Geometry check sheet. Reference: the model listing, model coordinates, mm. A direction names the side the tool comes from. Round coordinates to 2 decimals unless told otherwise and drop trailing zeros. Loops run counter-clockwise (first coordinate to the right, second up) from the corner with the lowest first, then second, coordinate; pieces in that order, holes last. Notation, with made-up numbers: (65, -6.5) - (98, -6.5) arc R14 ccw to (98, 20.5) - close; hole circle Ø4 at (49, 2.25). An arc over 180 degrees is marked (long way). Answer as CSV lines item,"result". Start each with the question number.
1) Cross-section at B-B on y = 27.5. Record the boundary of the cut face in (x, z).
2) Depth check by flat-ended pin: P1, Ø10, axis at y = 8.5, z = -25, coming from the +X side; P2, Ø3.5, axis at y = 14, z = 31, coming from the +X side; P3, Ø2, axis at x = -6.5, z = 17.5, coming from the +Y side; P4, Ø3.5, axis at x = 27, z = 22, coming from the +Y side. Enter the tip coordinate at first touch or a pass-through.
3) Cross-section at A-A on z = -22. State how many separate pieces and enclosed holes the cut face has, and give its area (3 significant figures).
4) Draft check along X on faces 1 (the cylindrical face through (-26.2, 1.23, 20.06)), 2 (the flat face through (0, 37, 30)), 3 (the flat face through (-29.98, 4.52, -29.87)). Enter one of: released by +X, released by -X, zero draft, split by the parting line, or undercut.
5) Cross-section at D-D on z = -1. Record the boundary of the cut face in (x, y), and give its area (3 significant figures).
6) Access from +Z, -Z, +X, -X, +Y, -Y to the whole of each face (thin tool, end or side, straight path). Record for faces 4 (the flat face through (13, 17, 39)), 5 (the flat face through (0, 36, 39)), 6 (the flat face through (0, 15, 20.65)), 7 (the flat face through (8, 15, 40)), 8 (the cylindrical face through (29.95, 4.27, -20.12)).
7) Thickness scan on line 1 along X through (y, z) = (0.65, -22); line 2 along Z through (x, y) = (-27, 1); line 3 along X through (y, z) = (9.5, 30). Record the ranges inside material, lowest first.
8) Cross-section at C-C on x = -19. Record the boundary of the cut face in (y, z).
from build123d import *

# Parameters (mm, degrees)
SKETCH1_R                          = 2.1
MAIN_CAP_EXTRUDE_DEPTH             = 6
MAIN_BODY_CHAMFER_SIZE             = 3
SKETCH4_R                          = 3.5
HOLE_COUNTERSINK_CUT_DEPTH         = 3
HOLE_COUNTERSINK_CHAMFER_SIZE      = 0.5
MAIN_PINION_CHIMNEY_EXTRUDE_DEPTH  = 32
SKETCH3_W                          = 28
SKETCH3_H                          = 24
PINION_CHIMNEY_CAP_EXTRUDE_DEPTH   = 5
INTERNAL_CHIMNEY_CHAMFER_SIZE      = 1
MAIN_CHIMNEY_EXTERNAL_CHAMFER_SIZE = 6
CHIMNEY_PLATE_CHAMFER_SIZE         = 8
CHIMNEY_FRONT_CHAMFER_SIZE         = 2


with BuildPart() as part:
    # Sketch1 → Main Cap Extrude (new body)
    with BuildSketch(Plane(origin=(0, 0, 0), x_dir=(1, 0, 0), z_dir=(0, 1, 0))):
        Polygon((-35, 27), (-27, 35), (27, 35), (35, 27), (35, -32), (27, -40), (5.5, -40), (5.5, -27.857106781), (9.5, -23.857106781), (9.5, -20.65), (-9.5, -20.65), (-9.5, -23.857106781), (-5.5, -27.857106781), (-5.5, -40), (-27, -40), (-35, -32), align=None)
        with Locations(Location((-27, 22, 0), (0, 0, 270))):
            Circle(SKETCH1_R, mode=Mode.SUBTRACT)
        with Locations(Location((27, 22, 0), (0, 0, 90))):
            Circle(SKETCH1_R, mode=Mode.SUBTRACT)
        with Locations(Location((27, -22, 0), (0, 0, 270))):
            Circle(SKETCH1_R, mode=Mode.SUBTRACT)
        with Locations(Location((-27, -22, 0), (0, 0, 90))):
            Circle(SKETCH1_R, mode=Mode.SUBTRACT)
    extrude(amount=MAIN_CAP_EXTRUDE_DEPTH)

    # Main Body Chamfer
    main_body_chamfer_edges = [part.edges().sort_by_distance(p)[0] for p in [
        (-31, 6, -31),
        (-35, 6, 2.5),
        (-31, 6, 36),
        (-16.25, 6, 40),
        (31, 6, -31),
        (16.25, 6, 40),
        (31, 6, 36),
        (35, 6, 2.5),
        (0, 6, -35),
    ]]
    chamfer(main_body_chamfer_edges, length=MAIN_BODY_CHAMFER_SIZE)

    # Sketch4 → Hole Countersink Cut (cut)
    with BuildSketch(Plane(origin=(0, 6, 0), x_dir=(1, 0, 0), z_dir=(0, 1, 0))):
        with Locations(Location((-27, 22, 0), (0, 0, 270))):
            Circle(SKETCH4_R)
        with Locations(Location((-27, -22, 0), (0, 0, 270))):
            Circle(SKETCH4_R)
        with Locations(Location((27, -22, 0), (0, 0, 270))):
            Circle(SKETCH4_R)
        with Locations(Location((27, 22, 0), (0, 0, 270))):
            Circle(SKETCH4_R)
    extrude(amount=-HOLE_COUNTERSINK_CUT_DEPTH, mode=Mode.SUBTRACT)

    # Hole Countersink Chamfer
    hole_countersink_chamfer_edges = [part.edges().sort_by_distance(p)[0] for p in [
        (27, 3, -19.9),
        (27, 6, -25.5),
        (27, 3, 19.9),
        (27, 6, 18.5),
        (-27, 3, 24.1),
        (-27, 6, 18.5),
        (-27, 3, -24.1),
        (-27, 6, -25.5),
    ]]
    chamfer(hole_countersink_chamfer_edges, length=HOLE_COUNTERSINK_CHAMFER_SIZE)

    # Sketch2 → Main Pinion Chimney Extrude (add)
    with BuildSketch(Plane(origin=(0, 0, 0), x_dir=(1, 0, 0), z_dir=(0, 1, 0))):
        Polygon((5.5, -27.857106781), (5.5, -40), (14, -40), (14, -16), (-14, -16), (-14, -40), (-5.5, -40), (-5.5, -27.857106781), (-9.5, -23.857106781), (-9.5, -20.65), (9.5, -20.65), (9.5, -23.857106781), align=None)
    extrude(amount=MAIN_PINION_CHIMNEY_EXTRUDE_DEPTH)

    # Sketch3 → Pinion Chimney Cap Extrude (add)
    with BuildSketch(Plane(origin=(0, 32, 0), x_dir=(1, 0, 0), z_dir=(0, 1, 0))):
        with Locations((0, -28)):
            Rectangle(SKETCH3_W, SKETCH3_H)
    extrude(amount=PINION_CHIMNEY_CAP_EXTRUDE_DEPTH)

    # Internal Chimney Chamfer
    internal_chimney_chamfer_edges = [part.edges().sort_by_distance(p)[0] for p in [
        (9.5, 32, 22.253553391),
        (7.5, 32, 25.857106781),
        (5.5, 32, 33.928553391),
        (-5.5, 32, 33.928553391),
        (-7.5, 32, 25.857106781),
        (-9.5, 32, 22.253553391),
        (0, 32, 20.65),
        (0, 32, 40),
        (-5.5, 16, 40),
        (5.5, 16, 40),
    ]]
    chamfer(internal_chimney_chamfer_edges, length=INTERNAL_CHIMNEY_CHAMFER_SIZE)

    # Main Chimney External Chamfer
    main_chimney_external_chamfer_edges = [part.edges().sort_by_distance(p)[0] for p in [
        (14, 21.5, 16),
        (-14, 21.5, 16),
        (-14, 37, 28),
        (14, 37, 28),
        (0, 37, 16),
    ]]
    chamfer(main_chimney_external_chamfer_edges, length=MAIN_CHIMNEY_EXTERNAL_CHAMFER_SIZE)

    # Chimney Plate Chamfer
    chimney_plate_chamfer_edges = [part.edges().sort_by_distance(p)[0] for p in [
        (-14, 6, 29.5),
        (0, 6, 16),
        (14, 6, 29.5),
        (11, 6, 19),
        (-11, 6, 19),
    ]]
    chamfer(chimney_plate_chamfer_edges, length=CHIMNEY_PLATE_CHAMFER_SIZE)

    # Chimney Front Chamfer
    chimney_front_chamfer_edges = [part.edges().sort_by_distance(p)[0] for p in [
        (14, 17, 40),
        (-14, 17, 40),
        (0, 37, 40),
        (11, 34, 40),
        (-11, 34, 40),
    ]]
    chamfer(chimney_front_chamfer_edges, length=CHIMNEY_FRONT_CHAMFER_SIZE)


solid = part.part
Answer block:
1,outline,"(-14, 22) - (-8, 16) - (8, 16) - (14, 22) - (14, 38) - (12, 40) - (6.5, 40) - (5.5, 39) - (5.5, 27.86) - (9.5, 23.86) - (9.5, 20.65) - (-9.5, 20.65) - (-9.5, 23.86) - (-5.5, 27.86) - (-5.5, 39) - (-6.5, 40) - (-12, 40) - (-14, 38) - close"
2,P1,"stops at x = 34.5"
2,P2,"stops at x = 15.73"
2,P3,"stops at y = 33.5"
2,P4,"passes through"
3,separate pieces,"3"
3,enclosed holes,"0"
3,area,"343 mm^2"
4,face 1,"undercut"
4,face 2,"zero draft"
4,face 3,"released by -X"
5,outline,"(-35, 0) - (35, 0) - (35, 3) - (32, 6) - (-32, 6) - (-35, 3) - close"
5,area,"411 mm^2"
6,face 4,"+Z, +X, +Y"
6,face 5,"+Z, +X, -X, +Y"
6,face 6,"-Y"
6,face 7,"+Z, +X, -X, +Y, -Y"
6,face 8,"+Y"
7,line 1,"x = -35 to -29.1, -24.9 to 24.9, 29.1 to 35"
7,line 2,"z = -35 to -24.1, -19.9 to 19.9, 24.1 to 40"
7,line 3,"x = -18.5 to -5.5, 5.5 to 18.5"
8,outline,"(0, -35) - (3, -35) - (6, -32) - (6, 15.69) - (9, 19.93) - (9, 34) - (3, 40) - (0, 40) - close"
